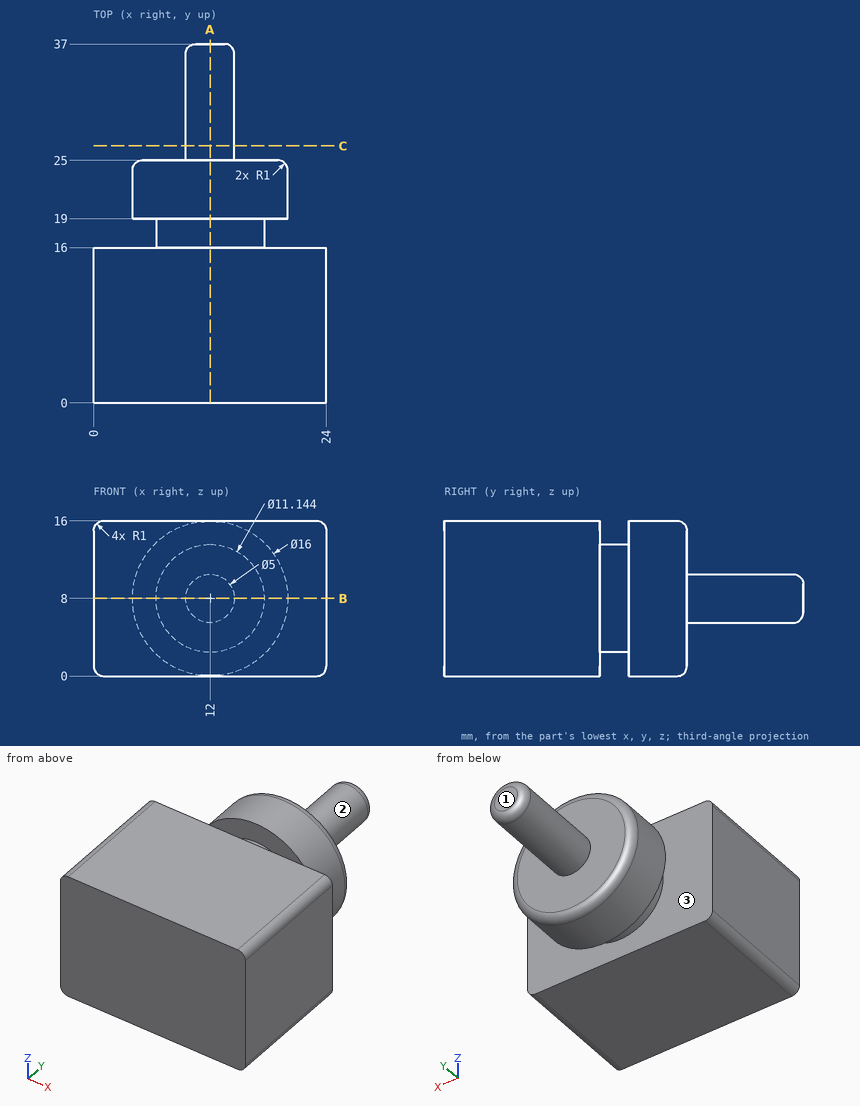
For this review, use the dimensioned drawing (mm, ordinates from the lowest corner) and the shaded views. A direction names the side the tool comes from. Round coordinates to 2 decimals unless told otherwise and drop trailing zeros. Loops run counter-clockwise (first coordinate to the right, second up) from the corner with the lowest first, then second, coordinate; pieces in that order, holes last. Notation, with made-up numbers: (-2.5, 59) -> (42.5, 59) arc R13 cw to (42.5, 79) -> close; hole circle Ø10 at (27, 19.5). An arc over 180 degrees is marked (long way). Write item = value, one per line. Start each with the question number.
Item 1: For the marked faces 1, 2 and 3, list the 3-axis set-ups (+Z, -Z, +X, -X, +Y, -Y) from which the entire face can be reached by the end or side of a thin tool; tool diameter is ignored.
Item 2: Take a section at C-C on y = 26.5. Give the boundary of the cut face in (x, z).
Item 3: Take a section at A-A on x = 12. Give the boundary of the cut face in (y, z).
Item 4: Take a section at B-B on z = 8. Give the boundary of the cut face in (x, y).
Item 5: To check wall thickness, follow L1, parallel to Y at x = 16.5, z = 11.75; L2, parallel to Y at x = 20.5, z = 9.75; L3, parallel to Y at x = 5, z = 5.5. State the ranges of each line that lie inside material, in increasing order.
Item 6: Insertion check: pin 1 (6 mm diameter, centred on x = 7, y = 21.5, fed in from -Z); pin 2 (2 mm diameter, centred on y = 23, z = 11.5, fed in from +X); pin 3 (3 mm diameter, centred on y = 31.5, z = 3, fed in from -X); pin 4 (10 mm diameter, centred on x = 2.5, y = 23.5, fed in from -Z) (1 decimal). Each pin has a flat end and moves straight along its axis. Give the tip position at first contact, or say it passes through.
Result:
q1.face_1 = +Z, -Z, +X, -X, +Y
q1.face_2 = +Y
q1.face_3 = none
q2.outline = circle Ø5 at (12, 8)
q3.outline = (0, 0) -> (16, 0) -> (16, 2.43) -> (19, 2.43) -> (19, 0) -> (24, 0) arc R1 ccw to (25, 1) -> (25, 5.5) -> (36, 5.5) arc R1 ccw to (37, 6.5) -> (37, 9.5) arc R1 ccw to (36, 10.5) -> (25, 10.5) -> (25, 15) arc R1 ccw to (24, 16) -> (19, 16) -> (19, 13.57) -> (16, 13.57) -> (16, 16) -> (0, 16) -> close
q4.outline = (0, 0) -> (24, 0) -> (24, 16) -> (17.57, 16) -> (17.57, 19) -> (20, 19) -> (20, 24) arc R1 ccw to (19, 25) -> (14.5, 25) -> (14.5, 36) arc R1 ccw to (13.5, 37) -> (10.5, 37) arc R1 ccw to (9.5, 36) -> (9.5, 25) -> (5, 25) arc R1 ccw to (4, 24) -> (4, 19) -> (6.43, 19) -> (6.43, 16) -> (0, 16) -> close
q5.L1 = 0 to 16, 19 to 25
q5.L2 = 0 to 16
q5.L3 = 0 to 16, 19 to 24.9
q6.pin_1 = 0.25
q6.pin_2 = 19.6
q6.pin_3 = through
q6.pin_4 = 1.4
